Geometry: final body of the model. Coordinates: model frame, mm. Round coordinates to 2 decimals unless told otherwise and drop trailing zeros. Loops run counter-clockwise (first coordinate to the right, second up) from the corner with the lowest first, then second, coordinate; pieces in that order, holes last. Notation, with made-up numbers: M 57,26 L 76,26 A28 ccw 76,48 Z; hole C -4,63 d7. An arc over 180 degrees is marked long. Answer as a JSON object with one key per item and string values.
from build123d import *


with BuildPart() as part:
    # Sweep1: sweep along a curve in space
    with BuildLine() as sweep1_path:
        Line((0, 0, 0), (0, 0, 45))
        ThreePointArc((0, 3, 48), (0, 0.878679656, 47.121320344), (0, 0, 45))
        Line((0, 3, 48), (0, 17, 48))
    # Sketch1 → Sweep1 (sweep)
    with BuildSketch(Plane(origin=(0, 0, 0), x_dir=(0, 1, 0), z_dir=(0, 0, 1))):
        Polygon((0.866025404, 0), (0.433012702, 0.75), (-0.433012702, 0.75), (-0.866025404, 0), (-0.433012702, -0.75), (0.433012702, -0.75), align=None)
    sweep(path=sweep1_path.line)


solid = part.part
1) Section query C-C (x = 0.25). Return the cut outline in (y, z), and give its area (3 significant figures).
Results:
{"outline": "M -0.72,0 L 0.72,0 L 0.72,45 A2.28 cw 3,47.28 L 17,47.28 L 17,48.72 L 3,48.72 A3.72 ccw -0.72,45 Z", "area": "92.0 mm2"}
2) Section query B-B (z = 32). Return the cut outline in (x, y), and give its area (3 significant figures).
Results:
{"outline": "M -0.75,-0.43 L 0,-0.87 L 0.75,-0.43 L 0.75,0.43 L 0,0.87 L -0.75,0.43 Z", "area": "1.95 mm2"}
3) Section query A-A (y = 3.5). Return the cut outline in (x, z).
Results:
{"outline": "M -0.75,47.57 L 0,47.13 L 0.75,47.57 L 0.75,48.43 L 0,48.87 L -0.75,48.43 Z"}
4) Ray query, line 1 (Y direction, x = -0.2, z = 30.5); line 2 (Y direction, x = -0.65, z = 5); line 3 (Z direction, x = 0.1, y = 8). Return the intervals inside material, ascending.
Results:
{"line 1": "-0.75 to 0.75", "line 2": "-0.49 to 0.49", "line 3": "47.19 to 48.81"}
